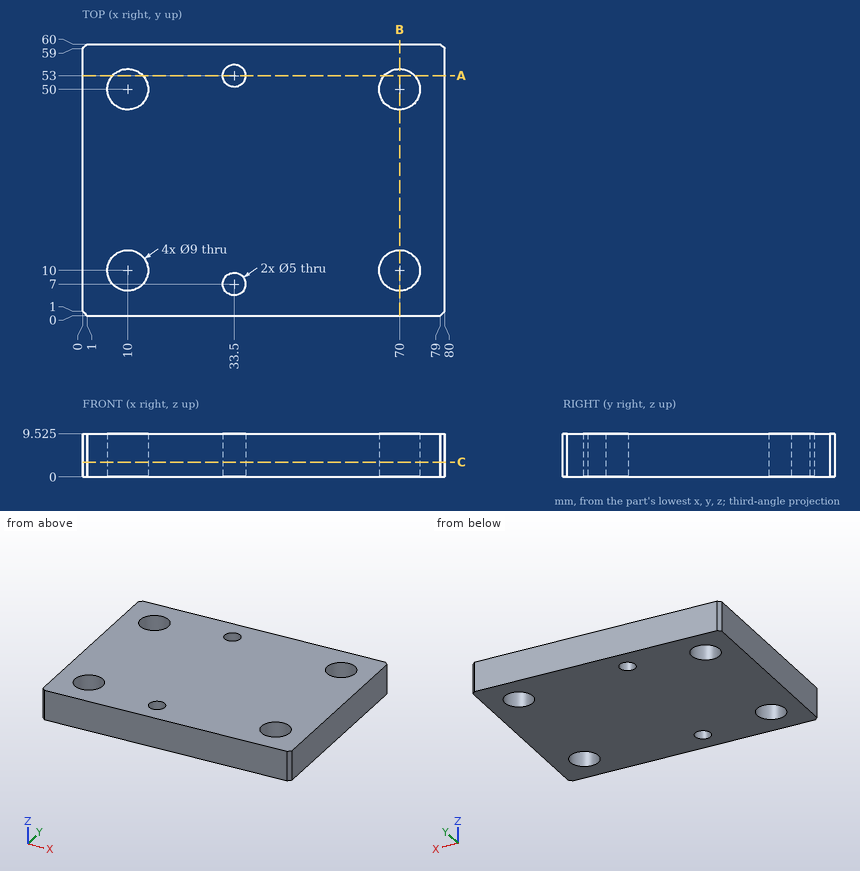
Design review of the part shown in the three views and the two pictorial views. Dimensions are in mm from the part's minimum x, y and z. Round coordinates to 2 decimals unless told otherwise and drop trailing zeros. Write each loop counter-clockwise with the first axis right and the second up, starting at its lowest first coordinate (ties: lowest second). Pieces come first, ordered by that corner, then holes.
1) For line 1 along Y through (x, z) = (70, 7.75); line 2 along Y through (x, z) = (33, 6.25), list the stretches that pass through material, from the lowest coordinate up.
Answer below:
line 1: y = 0 to 5.5, 14.5 to 45.5, 54.5 to 60
line 2: y = 0 to 4.55, 9.45 to 50.55, 55.45 to 60
2) Take a section at A-A on y = 53. Give the boundary of the cut face in (x, z) (3 decimals).
Answer below:
outline: (0, 0) - (6.646, 0) - (6.646, 9.525) - (0, 9.525) - close; (13.354, 0) - (31, 0) - (31, 9.525) - (13.354, 9.525) - close; (36, 0) - (66.646, 0) - (66.646, 9.525) - (36, 9.525) - close; (73.354, 0) - (80, 0) - (80, 9.525) - (73.354, 9.525) - close
3) Take a section at B-B on x = 70. Give the boundary of the cut face in (y, z) (3 decimals).
Answer below:
outline: (0, 0) - (5.5, 0) - (5.5, 9.525) - (0, 9.525) - close; (14.5, 0) - (45.5, 0) - (45.5, 9.525) - (14.5, 9.525) - close; (54.5, 0) - (60, 0) - (60, 9.525) - (54.5, 9.525) - close
4) Take a section at C-C on z = 3.25. Give the boundary of the cut face in (x, y).
Answer below:
outline: (0, 1) - (1, 0) - (79, 0) - (80, 1) - (80, 59) - (79, 60) - (1, 60) - (0, 59) - close; hole circle Ø9 at (10, 10); hole circle Ø9 at (10, 50); hole circle Ø5 at (33.5, 7); hole circle Ø5 at (33.5, 53); hole circle Ø9 at (70, 10); hole circle Ø9 at (70, 50)
5) Insertion check: pin 1 Ø7 at (x, y) = (10, 50) entering from -Z. The pin has a flat end and moves straight along its axis. Give the tip position at first contact, or say it passes through.
Answer below:
pin 1: passes through
